Work out the finished part from the listing and answer in its coordinate system (mm). Face numbers are marked on the shaded views. Coordinates: 2 decimals unless noted, no trailing zeros. Write each loop counter-clockwise with the first axis right and the second up, starting at its lowest first coordinate (ties: lowest second). Pieces come first, ordered by that corner, then holes. Notation, with made-up numbers: M 68,-22.5 L 122,-22.5 A34 cw 122,11.5 Z; hole C 17.5,50.5 d7. An arc over 180 degrees is marked long. Use CSV: the item, a comma, the result in double quotes.
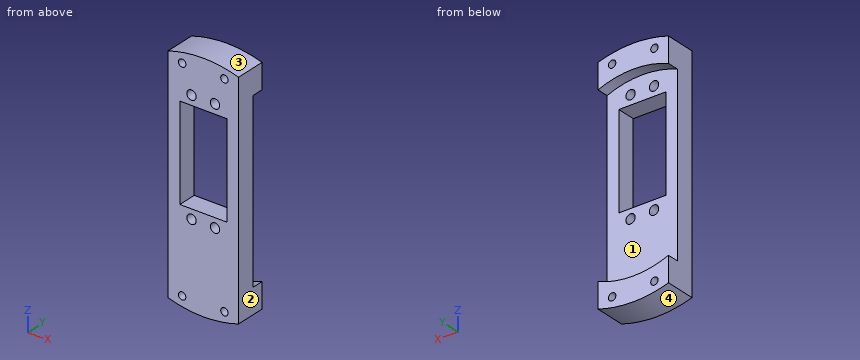
from build123d import *

# Parameters (mm, degrees)
SKETCH_1_R                  = 2
SKETCH_1_W                  = 20
SKETCH_1_H                  = 40
EXTRUDE_1_DEPTH             = 8
EXTRUDE_2_DEPTH             = 5
HOLE_WIZARD_M31_D           = 3.15
PATTERN_LINEAR_1_COUNT      = 2
PATTERN_LINEAR_1_PITCH      = 18
PATTERN_LINEAR_1_COUNT_DIR2 = 2
PATTERN_LINEAR_1_PITCH_DIR2 = 90


with BuildPart() as part:
    # Эскиз1 → Бобышка-Вытянуть1 (new body)
    with BuildSketch(Plane(origin=(0, 0, 0), x_dir=(1, 0, 0), z_dir=(0, 1, 0))):
        with BuildLine():
            Line((-15, -47.696960071), (-15, 47.696960071))
            ThreePointArc((-15, 47.696960071), (0, 50), (15, 47.696960071))
            Line((15, 47.696960071), (15, -47.696960071))
            ThreePointArc((15, -47.696960071), (0, -50), (-15, -47.696960071))
        make_face()
        with Locations(Location((-5, -34, 0), (0, 0, 270))):
            Circle(SKETCH_1_R, mode=Mode.SUBTRACT)
        with Locations(Location((5, -34, 0), (0, 0, 90))):
            Circle(SKETCH_1_R, mode=Mode.SUBTRACT)
        with Locations(Location((5, 14, 0), (0, 0, 270))):
            Circle(SKETCH_1_R, mode=Mode.SUBTRACT)
        with Locations(Location((-5, 14, 0), (0, 0, 90))):
            Circle(SKETCH_1_R, mode=Mode.SUBTRACT)
        with Locations((0, -10)):
            Rectangle(SKETCH_1_W, SKETCH_1_H, mode=Mode.SUBTRACT)
    extrude(amount=EXTRUDE_1_DEPTH)

    # Эскиз2 → Бобышка-Вытянуть2 (add)
    with BuildSketch(Plane(origin=(0, 8, 0), x_dir=(1, 0, 0), z_dir=(0, 1, 0))):
        with BuildLine():
            Line((-15, 37.080992435), (-15, 47.696960071))
            ThreePointArc((-15, 47.696960071), (0, 50), (15, 47.696960071))
            Line((15, 47.696960071), (15, 37.080992435))
            ThreePointArc((15, 37.080992435), (0, 40), (-15, 37.080992435))
        make_face()
        with BuildLine():
            Line((-15, -37.080992435), (-15, -47.696960071))
            ThreePointArc((-15, -47.696960071), (0, -50), (15, -47.696960071))
            Line((15, -47.696960071), (15, -37.080992435))
            ThreePointArc((15, -37.080992435), (0, -40), (-15, -37.080992435))
        make_face()
    extrude(amount=EXTRUDE_2_DEPTH)

    # Сверло под метчик  спиральное M31 (through all)
    with Locations(Plane(origin=(0, 13, 0), x_dir=(1, 0, 0), z_dir=(0, 1, 0))):
        with Locations((-9, -45)):
            hole_wizard_m31 = Hole(HOLE_WIZARD_M31_D / 2)

    # Линейный массив1: Hole Wizard M31 2 × 2
    with Locations(*[(i * PATTERN_LINEAR_1_PITCH, 0, -j * PATTERN_LINEAR_1_PITCH_DIR2) for i in range(PATTERN_LINEAR_1_COUNT) for j in range(PATTERN_LINEAR_1_COUNT_DIR2) if (i, j) != (0, 0)]):
        add(hole_wizard_m31, mode=Mode.SUBTRACT)


solid = part.part
Item 1: The part is cut by section A-A (z = 28.5). Write down the section's boundary in (x, y).
Answer:
outline,"M -15,0 L -10,0 L -10,8 L -15,8 Z; M 10,0 L 15,0 L 15,8 L 10,8 Z"
Item 2: Consider probe 1 along X at (y, z) = (4.5, 45) (3 decimals); probe 2 along X at (y, z) = (3.5, -14); probe 3 along Z at (x, y) = (4.5, 4.5). Determine where each line is inside the solid, lowest interval first.
Answer:
probe 1,"x = -15 to -10.575, -7.425 to 7.425, 10.575 to 15"
probe 2,"x = -15 to -7, -3 to 3, 7 to 15"
probe 3,"z = -49.8 to -15.94, -12.06 to -10, 30 to 32.06, 35.94 to 49.8"
Item 3: The part is cut by section D-D (x = 9). Write down the section's boundary in (y, z) (3 decimals).
Answer:
outline,"M 0,-49.183 L 13,-49.183 L 13,-46.575 L 0,-46.575 Z; M 0,-43.425 L 13,-43.425 L 13,-38.974 L 8,-38.974 L 8,-10 L 0,-10 Z; M 0,30 L 8,30 L 8,38.974 L 13,38.974 L 13,43.425 L 0,43.425 Z; M 0,46.575 L 13,46.575 L 13,49.183 L 0,49.183 Z"
Item 4: The part is cut by section C-C (y = 6.75). Count the separate pieces of the cut face and the enclosed holes in it, then the cut area to 3 significant figures.
Answer:
separate pieces,"1"
enclosed holes,"9"
area,"2,070 mm2"
Item 5: For a pull along Z with two mould halves and no side action, classify the marked faces 1, 2, 3 and 4 as released by +Z, released by -Z, zero draft, split by the parting line, or undercut.
Answer:
face 1,"undercut"
face 2,"zero draft"
face 3,"released by +Z"
face 4,"released by -Z"
Item 6: The part is cut by section B-B (z = -14). Write down the section's boundary in (x, y), then the cut area to 3 significant figures.
Answer:
outline,"M -15,0 L -7,0 L -7,8 L -15,8 Z; M -3,0 L 3,0 L 3,8 L -3,8 Z; M 7,0 L 15,0 L 15,8 L 7,8 Z"
area,"176 mm2"
Item 7: Given pin 1 (2 mm diameter, centred on x = 10.5, y = 7.5, fed in from -Z); pin 2 (2.5 mm diameter, centred on x = 5, z = -14, fed in from -Y); pin 3 (1 mm diameter, centred on x = 6.5, y = 6, fed in from +Z); pin 4 (1 mm diameter, centred on x = 6.5, y = 4, fed in from -Z), each flat-ended and moving along its own axis, determine where each tip first touches the part or whether it passes through.
Answer:
pin 1,"stops at z = -49.09"
pin 2,"passes through"
pin 3,"stops at z = 49.64"
pin 4,"stops at z = -49.64"
